```python
from build123d import *

# Parameters (mm, degrees)
F0_W     = 5
F0_H     = 50
F0_W_2   = 4
F0_H_2   = 3
F1_DEPTH = 10
F3_R     = 3
F4_DEPTH = 10


with BuildPart() as f1:
    # F0 (on Top) → F1 (new body)
    with BuildSketch(Plane.XY):
        with Locations((-2.5, -25)):
            Rectangle(F0_W, F0_H)
        Polygon((-5, 0), (0, 0), (0, 7), (-80, 7), (-80, 0), (-75.83991, 0), (-44.478558, 0), (-40, 0), align=None)
        Polygon((0, 7), (0, 0), (28, 0), (32, 0), (32, 7), align=None)
        with Locations((30, -1.5)):
            Rectangle(F0_W_2, F0_H_2)
        Polygon((-61.87452, -48.874639), (-40, 0), (-44.478558, 0), (-63.619636, -42.76726), align=None)
        Polygon((32, -3), (28, -3), (17, -3), (17, -7), (32, -7), align=None)
        Polygon((-56.921913, -66.207265), (-61.87452, -48.874639), (-63.619636, -42.76726), (-75.83991, 0), (-80, 0), (-60.767984, -67.306237), align=None)
    extrude(amount=F1_DEPTH)

    # F3 (on face) → F4 (cut)
    with BuildSketch(Plane(origin=(-73.961299, -21.133627, 0), x_dir=(0.274743, -0.961518, 0), z_dir=(-0.961518, -0.274743, 0))):
        with Locations((39.963152, 5.025908)):
            Circle(F3_R)
    extrude(amount=-F4_DEPTH, mode=Mode.SUBTRACT)


solid = f1.part
```
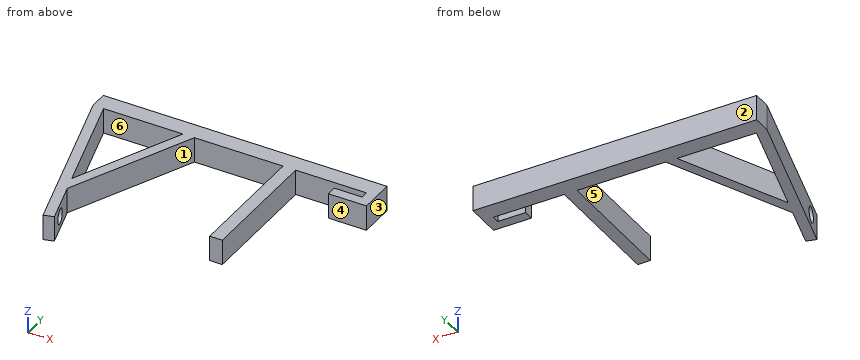
Geometry check sheet. Reference: the model listing, model coordinates, mm. Face numbers are marked on the shaded views. A direction names the side the tool comes from. Give positions to 0.01 mm unless a question says otherwise; leave off trailing zeros. Write each loop counter-clockwise with the first axis right and the second up, starting at its lowest first coordinate (ties: lowest second). Pieces come first, ordered by that corner, then holes. Notation, with made-up numbers: (78, 67.5) -> (97, 67.5) arc R24 cw to (97, 102.5) -> close; hole circle Ø8 at (27, -25.5). An arc over 180 degrees is marked (long way). Use one line per item in the form item = value.
Item 1: Depth check by flat-ended pin: pin 1 Ø6 at (x, z) = (-1, 1) entering from -Y; pin 2 Ø5 at (y, z) = (-12.5, 5) entering from -X; pin 3 Ø4 at (x, y) = (-46.5, -1) entering from +Z; pin 4 Ø5 at (x, z) = (-37, 5.5) entering from -Y. Enter the tip coordinate at first touch or a pass-through.
Results list:
pin_1 = -50
pin_2 = -77.14
pin_3 = 10
pin_4 = 0
Item 2: Access from +Z, -Z, +X, -X, +Y, -Y to the whole of each face (thin tool, end or side, straight path). Record for the marked faces 4, 5 and 6.
Results list:
face_4 = +Z, -Z, +X, -Y
face_5 = +Z, -Z, -Y
face_6 = +Z, -Z
Item 3: Sectioned sample at B-B on y = -31. Enter the section's corners in (x, z).
Results list:
outline = (-71.14, 0) -> (-66.98, 0) -> (-66.98, 10) -> (-71.14, 10) -> close; (-58.35, 0) -> (-53.87, 0) -> (-53.87, 10) -> (-58.35, 10) -> close; (-5, 0) -> (0, 0) -> (0, 10) -> (-5, 10) -> close
Item 4: Mould release check, pull along X, two halves, no side actions. Record for the marked faces 1, 2 and 3: released by +X, released by -X, zero draft, split by the parting line, or undercut.
Results list:
face_1 = undercut
face_2 = zero draft
face_3 = released by +X
Item 5: Sectioned sample at C-C on x = -18.5. Enter the section's corners in (y, z).
Results list:
outline = (0, 0) -> (7, 0) -> (7, 10) -> (0, 10) -> close
Item 6: Scan lines: line 1 (Y direction, x = 21, z = 2.5); line 2 (X direction, y = -13, z = 1.75); line 3 (X direction, y = -15, z = 3.25). Record each from-to range of solid material in increasing order.
Results list:
line_1 = -7 to -3, 0 to 7
line_2 = -76.29 to -72.13, -50.3 to -45.82, -5 to 0
line_3 = -75.71 to -71.55, -51.19 to -46.71, -5 to 0
Item 7: Sectioned sample at D-D on x = -2. Enter the section's corners in (y, z).
Results list:
outline = (-50, 0) -> (7, 0) -> (7, 10) -> (-50, 10) -> close
Item 8: Sectioned sample at A-A on x = -47. Enter the section's corners in (y, z), plus the area to 3 significant figures.
Results list:
outline = (-15.64, 0) -> (-5.63, 0) -> (-5.63, 10) -> (-15.64, 10) -> close; (0, 0) -> (7, 0) -> (7, 10) -> (0, 10) -> close
area = 170 mm2
